The drawing under review shows one solid part. Ordinate dimensions are in mm from its lowest x, y, z. Round coordinates to 2 decimals unless told otherwise and drop trailing zeros. Write each loop counter-clockwise with the first axis right and the second up, starting at its lowest first coordinate (ties: lowest second). Pieces come first, ordered by that corner, then holes. Notation, with made-up numbers: (46.5, 19) -> (102.5, 19) arc R18 cw to (102.5, 46) -> close; hole circle Ø1 at (40.25, 48). An arc over 180 degrees is marked (long way). Answer in a Markdown table with one row per item. Add a question column.
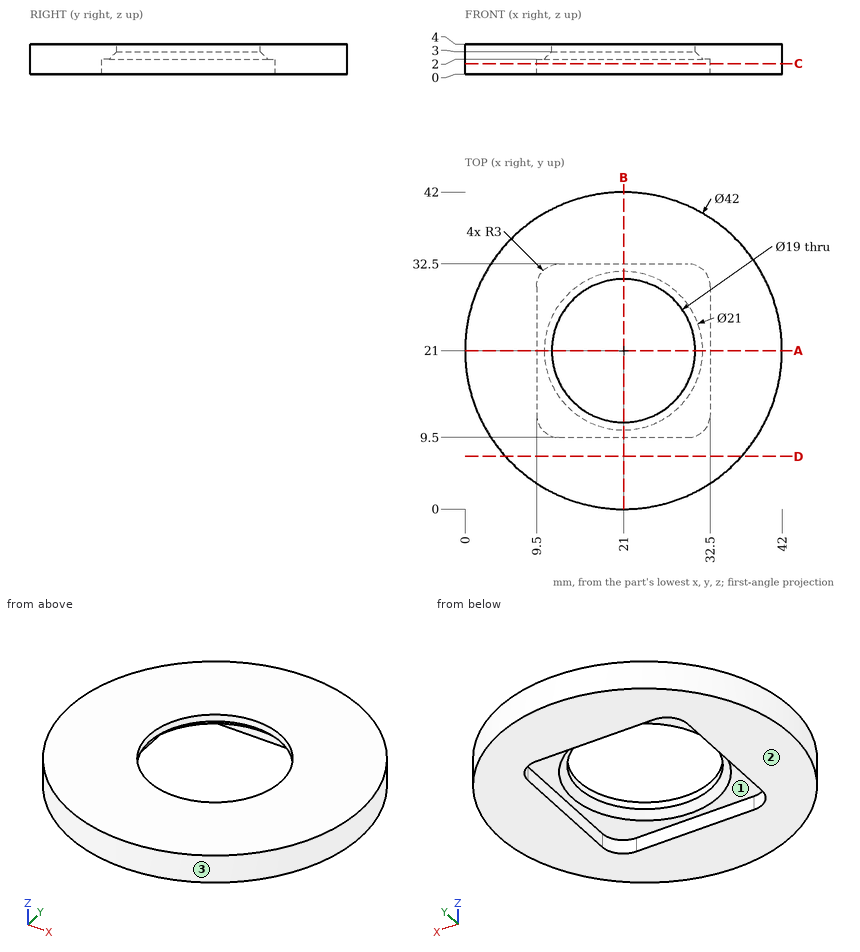
1. Add section D-D on y = 7. Write out the cut boundary in (x, z), plus the area to 3 significant figures.
2. Add section C-C on z = 1.4. Write out the cut boundary in (x, y).
3. Insertion check: pin 1 Ø2 at (x, z) = (21, 3.5) entering from -Y; pin 2 Ø2 at (x, z) = (25, 1) entering from +Y; pin 3 Ø5 at (x, y) = (22.5, 31.5) entering from -Z; pin 4 Ø1 at (y, z) = (18.5, 1) entering from +X. Each pin has a flat end and moves straight along its axis. Give the tip position at first contact, or say it passes through.
4. Mouldability with a two-part tool opening along X and no side actions: class the marked faces 1, 2 and 3 as pulls with the +X half, pulls with the -X half, needs draft (parallel to the pull), parting line crosses it, or undercut.
5. Add section A-A on y = 21. Write out the cut boundary in (x, z).
6. For L1, parallel to Y at x = 21, z = 3.5; L2, parallel to X at y = 29.5, z = 1, list the stretches that pass through material, from the lowest coordinate up.
Filled in:
| question | item | result |
|---|---|---|
| 1 | outline | (5.35, 0) -> (36.65, 0) -> (36.65, 4) -> (5.35, 4) -> close |
| 1 | area | 125 mm² |
| 2 | outline | circle Ø42 at (21, 21); hole (9.5, 12.5) arc R3 ccw to (12.5, 9.5) -> (29.5, 9.5) arc R3 ccw to (32.5, 12.5) -> (32.5, 29.5) arc R3 ccw to (29.5, 32.5) -> (12.5, 32.5) arc R3 ccw to (9.5, 29.5) -> close |
| 3 | pin 1 | y = 0 |
| 3 | pin 2 | y = 41.78 |
| 3 | pin 3 | z = 0 |
| 3 | pin 4 | x = 41.9 |
| 4 | face 1 | undercut |
| 4 | face 2 | needs draft |
| 4 | face 3 | parting line crosses it |
| 5 | outline | (0, 0) -> (9.5, 0) -> (9.5, 2) -> (10.5, 2) -> (11.5, 3) -> (11.5, 4) -> (0, 4) -> close; (30.5, 3) -> (31.5, 2) -> (32.5, 2) -> (32.5, 0) -> (42, 0) -> (42, 4) -> (30.5, 4) -> close |
| 6 | L1 | 0 to 11.5, 30.5 to 42 |
| 6 | L2 | 1.8 to 9.5, 32.5 to 40.2 |
